Job drawing, mm, ordinate dimensions from the low corner. One solid piece. A direction names the side the tool comes from. Give positions to 0.01 mm unless a question says otherwise; leave off trailing zeros. Write each loop counter-clockwise with the first axis right and the second up, starting at its lowest first coordinate (ties: lowest second). Pieces come first, ordered by that corner, then holes. Notation, with made-up numbers: (46.5, 67) - (63.5, 67) arc R26 ccw to (63.5, 101) - close; hole circle Ø2 at (14.25, 55.25). An arc over 180 degrees is marked (long way). Answer in a Markdown table with one row per item. Add a question column.
1. Which spindle directions (+Z, -Z, +X, -X, +Y, -Y) get a long thin tool onto all of the face, cutting with end or side? Do the marked faces 4, 5, 6 and 7. Say none if no direction does.
2. Band-saw the part on C-C on y = 32.5. Write the cut outline in (x, z), plus the area to 3 significant figures.
3. Drop flat-ended pins along their axis: pin 1 Ø6 at (x, y) = (34.5, 9.5) entering from +Z; pin 2 Ø3 at (x, z) = (23, 5) entering from +Y; pin 3 Ø6 at (x, y) = (87, 30) entering from +Z; pin 4 Ø10 at (x, y) = (24.5, 22.5) entering from -Z. Give the stop position or say it passes through.
4. Probe line 1 along Y through (x, z) = (83, 13); line 2 along Y through (x, z) = (33.5, 18); line 3 along X through (y, z) = (26, 16). List the from-to ranges inside material, lowest first.
5. Band-saw the part on D-D on y = 25. Write the cut outline in (x, z).
6. Band-saw the part on A-A on z = 14.5. Write the cut outline in (x, y), plus the area to 3 significant figures.
7. Band-saw the part on B-B on x = 38.5. Write the cut outline in (y, z), plus the area to 3 significant figures.
8. Pull direction Y, two halves, no side cores. Call the marked faces 1, 2 and 3: released by +Y, released by -Y, zero draft, split by the parting line, or undercut.
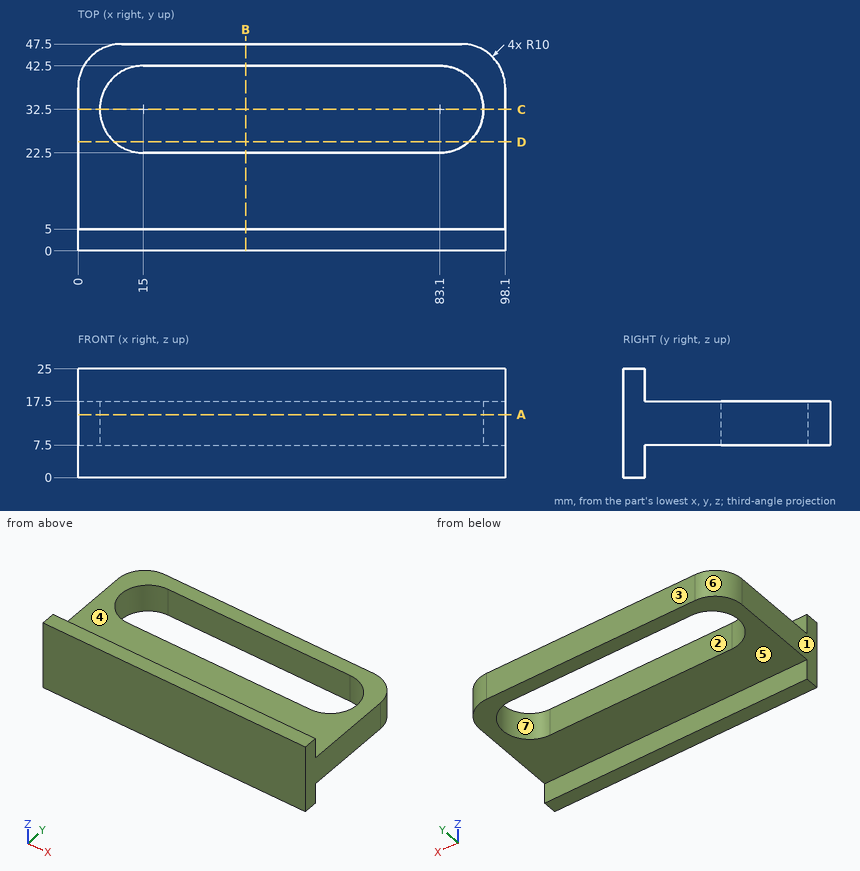
Values:
| question | item | result |
|---|---|---|
| 1 | face 4 | +Z, +X, -X, +Y |
| 1 | face 5 | -Z, +X, -X, +Y |
| 1 | face 6 | +Z, -Z, -X, +Y |
| 1 | face 7 | +Z, -Z |
| 2 | outline | (0, 7.5) - (5, 7.5) - (5, 17.5) - (0, 17.5) - close; (93.1, 7.5) - (98.1, 7.5) - (98.1, 17.5) - (93.1, 17.5) - close |
| 2 | area | 100 mm² |
| 3 | pin 1 | stops at z = 17.5 |
| 3 | pin 2 | stops at y = 5 |
| 3 | pin 3 | passes through |
| 3 | pin 4 | stops at z = 7.5 |
| 4 | line 1 | y = 0 to 22.5, 42.5 to 47.5 |
| 4 | line 2 | y = 0 to 5 |
| 4 | line 3 | x = 0 to 7.4, 90.7 to 98.1 |
| 5 | outline | (0, 7.5) - (8.39, 7.5) - (8.39, 17.5) - (0, 17.5) - close; (89.71, 7.5) - (98.1, 7.5) - (98.1, 17.5) - (89.71, 17.5) - close |
| 6 | outline | (0, 0) - (98.1, 0) - (98.1, 37.5) arc R10 ccw to (88.1, 47.5) - (10, 47.5) arc R10 ccw to (0, 37.5) - close; hole (15, 22.5) - (83.1, 22.5) arc R10 ccw to (83.1, 42.5) - (15, 42.5) arc R10 ccw to start |
| 6 | area | 2,940 mm² |
| 7 | outline | (0, 0) - (5, 0) - (5, 7.5) - (22.5, 7.5) - (22.5, 17.5) - (5, 17.5) - (5, 25) - (0, 25) - close; (42.5, 7.5) - (47.5, 7.5) - (47.5, 17.5) - (42.5, 17.5) - close |
| 7 | area | 350 mm² |
| 8 | face 1 | zero draft |
| 8 | face 2 | undercut |
| 8 | face 3 | released by +Y |
